from build123d import *

# Parameters (mm, degrees)
CROQUIS1_W              = 37.5
CROQUIS1_H              = 14
SALIENTE_EXTRUIR1_DEPTH = 15.5
CROQUIS2_W              = 17
CROQUIS2_H              = 10
SALIENTE_EXTRUIR2_DEPTH = 8
CROQUIS3_R              = 1.6
CORTAR_EXTRUIR1_DEPTH   = 107.526693573
CORTAR_EXTRUIR2_DEPTH   = 108.142287781


with BuildPart() as part:
    # Croquis1 → Saliente-Extruir1 (new, symmetric)
    with BuildSketch(Plane.XY):
        Polygon((-91.394558809, -11.557384804), (-91.394558809, -29.877384804), (-37.5, -7), (-37.5, 7), align=None)
        Polygon((37.5, 7), (91.394558809, -11.557384804), (91.394558809, -29.877384804), (37.5, -7), align=None)
        with Locations((18.75, 0)):
            Rectangle(CROQUIS1_W, CROQUIS1_H)
        with Locations((-18.75, 0)):
            Rectangle(CROQUIS1_W, CROQUIS1_H)
    extrude(amount=SALIENTE_EXTRUIR1_DEPTH, both=True)

    # Croquis2 → Saliente-Extruir2 (add)
    with BuildSketch(Plane.ZY.offset(91.394558809)):
        with Locations((0, -20.717384804)):
            Rectangle(CROQUIS2_W, CROQUIS2_H)
    saliente_extruir2 = extrude(amount=SALIENTE_EXTRUIR2_DEPTH)

    # Croquis3 → Cortar-Extruir1 (cut, through all)
    with BuildSketch(Plane.XY.offset(8.5)):
        with Locations((-95.394558809, -20.717384804)):
            Circle(CROQUIS3_R)
    cortar_extruir1 = extrude(amount=-CORTAR_EXTRUIR1_DEPTH, mode=Mode.SUBTRACT)

    # Simetría1: Saliente-Extruir2, Cortar-Extruir1 across plane
    add(saliente_extruir2.mirror(Plane(origin=(0, 0, 0), x_dir=(0, 0, 1), z_dir=(1, 0, 0))))
    add(cortar_extruir1.mirror(Plane(origin=(0, 0, 0), x_dir=(0, 0, 1), z_dir=(1, 0, 0))), mode=Mode.SUBTRACT)

    # Croquis4 → Cortar-Extruir2 (cut, through all)
    with BuildSketch(Plane(origin=(0, 7, 0), x_dir=(1, 0, 0), z_dir=(0, 1, 0))):
        Polygon((-8.675, 12.5), (8.675, 12.5), (10.015331351, 10.33066557), (1.135565493, -7.02), (-1.544434507, -7.02), (-10.015331351, 10.33066557), align=None)
        Polygon((3.8246, -12.5), (2.484268649, -10.33066557), (10.955165493, 7.02), (13.635165493, 7.02), (22.514931351, -10.33066557), (21.1746, -12.5), align=None)
        Polygon((35.015331351, 10.33066557), (26.135565493, -7.02), (23.455565493, -7.02), (14.984668649, 10.33066557), (16.325, 12.5), (33.675, 12.5), align=None)
        Polygon((28.8246, -12.5), (27.484268649, -10.33066557), (35.955165493, 7.02), (38.635165493, 7.02), (47.514931351, -10.33066557), (46.1746, -12.5), align=None)
        Polygon((60.015331351, 10.33066557), (51.135565493, -7.02), (48.455565493, -7.02), (39.984668649, 10.33066557), (41.325, 12.5), (58.675, 12.5), align=None)
        Polygon((53.8246, -12.5), (52.484268649, -10.33066557), (60.955165493, 7.02), (63.635165493, 7.02), (72.514931351, -10.33066557), (71.1746, -12.5), align=None)
        Polygon((85.015331351, 10.33066557), (76.135565493, -7.02), (73.455565493, -7.02), (64.984668649, 10.33066557), (66.325, 12.5), (83.675, 12.5), align=None)
        Polygon((78.8246, -12.5), (77.484268649, -10.33066557), (85.955165493, 7.02), (85.955165493, -12.5), align=None)
        Polygon((-3.8246, -12.5), (-2.484268649, -10.33066557), (-10.955165493, 7.02), (-13.635165493, 7.02), (-22.514931351, -10.33066557), (-21.1746, -12.5), align=None)
        Polygon((-83.675, 12.5), (-85.015331351, 10.33066557), (-76.135565493, -7.02), (-73.455565493, -7.02), (-64.984668649, 10.33066557), (-66.325, 12.5), align=None)
        Polygon((-60.955165493, 7.02), (-63.635165493, 7.02), (-72.514931351, -10.33066557), (-71.1746, -12.5), (-53.8246, -12.5), (-52.484268649, -10.33066557), align=None)
        Polygon((-58.675, 12.5), (-60.015331351, 10.33066557), (-51.135565493, -7.02), (-48.455565493, -7.02), (-39.984668649, 10.33066557), (-41.325, 12.5), align=None)
        Polygon((-35.955165493, 7.02), (-38.635165493, 7.02), (-47.514931351, -10.33066557), (-46.1746, -12.5), (-28.8246, -12.5), (-27.484268649, -10.33066557), align=None)
        Polygon((-33.675, 12.5), (-35.015331351, 10.33066557), (-26.135565493, -7.02), (-23.455565493, -7.02), (-14.984668649, 10.33066557), (-16.325, 12.5), align=None)
        Polygon((-85.955165493, 7.02), (-85.955165493, -12.5), (-78.8246, -12.5), (-77.484268649, -10.33066557), align=None)
    extrude(amount=-CORTAR_EXTRUIR2_DEPTH, mode=Mode.SUBTRACT)


solid = part.part
Build history of the part. All positions in model axes, mm. A direction names the side the tool comes from. Round coordinates to 2 decimals unless told otherwise and drop trailing zeros. Answer as a JSON object with one key per item and string values. Group by question number.
(1) Mould opens along Z. For faces 1 (the flat face through (70.81, -21.14, 3.66)), 2 (the flat face through (18.01, 0.1, 1.53)) say: pulls with the +Z half, pulls with the -Z half, needs draft (parallel to the pull), parting line crosses it, or undercut.
(2) Which spindle directions (+Z, -Z, +X, -X, +Y, -Y) get a long thin tool onto all of the face, cutting with end or side? Do faces 3 (the flat face through (95, -15.717, 0)), 4 (the flat face through (-8.9, -7, -3.2)), 5 (the flat face through (-82, -17, 12.5)), 6 (the flat face through (99.395, -21, 0)), 7 (the flat face through (-95, -25.717, 0)). Say none if no direction does.
(3) Drill centre lines: L1, parallel to Z at x = 39, y = -4; L2, parallel to Z at x = -59.5, y = -4.5; L3, parallel to X at y = -16.5, z = -2. Where is each one in solid material? Low to high.
(4) Flat gauge pins, fed straight in: pin 1 (4 mm diameter, centred on x = 69.5, z = -5, fed in from -Y); pin 2 (2.5 mm diameter, centred on x = 94.5, z = -2.5, fed in from -Y). Where does each tip first touch, or does it go through?
(5) Cut at A-A (z = 2). Give the number of separate pieces and of enclosed holes in the cut face, and give its area (3 significant figures).
Responses:
{
 "1": {"face 1": "needs draft", "face 2": "undercut"},
 "2": {"face 3": "+Z, -Z, +X, +Y", "face 4": "+Z, -Z, -Y", "face 5": "+Y, -Y", "face 6": "+Z, -Z, +X, +Y, -Y", "face 7": "+Z, -Z, -X, -Y"},
 "3": {"L1": "z = -15.5 to -6.31, 12.5 to 15.5", "L2": "z = -15.5 to -11.16, -9.32 to -4.04, 12.5 to 15.5", "L3": "x = -99.39 to -85.96, -83.5 to -80.75, -69.05 to -66.2, 66.2 to 69.05, 80.75 to 83.5, 85.96 to 99.39"},
 "4": {"pin 1": "stops at y = -20.12", "pin 2": "stops at y = -25.72"},
 "5": {"separate pieces": "16", "enclosed holes": "2", "area": "932 mm2"}
}
